Design review of the part built by this model. Coordinates are the model's own, in mm. A direction names the side the tool comes from. Give positions to 0.01 mm unless a question says otherwise; leave off trailing zeros. Write each loop counter-clockwise with the first axis right and the second up, starting at its lowest first coordinate (ties: lowest second). Pieces come first, ordered by that corner, then holes. Notation, with made-up numbers: (-2.5, 65) -> (18.5, 65) arc R33 ccw to (18.5, 100) -> close; hole circle Ø6 at (30.5, 66). An arc over 180 degrees is marked (long way). Return JSON: item names as keys, results as strings. Group by question number.
from build123d import *

# Parameters (mm, degrees)
F1_DEPTH = 10
F3_START = -8.5
F3_DEPTH = 1.5
F4_W     = 100
F4_H     = 3.1556577078
F5_DEPTH = 15
F6_R     = 2.1
F7_DEPTH = 3.1556577078


with BuildPart() as f1:
    # F0 (on Front) → F1 (new body)
    with BuildSketch(Plane.XZ):
        with BuildLine():
            Line((-40, 0), (0, 0))
            Line((0, 0), (40, 0))
            Line((40, 0), (39, 3))
            Line((39, 3), (7.4807440028, 74.4629067455))
            ThreePointArc((7.4807440028, 74.4629067455), (5.4899088977, 80.1098826107), (0, 82.5))
            ThreePointArc((0, 82.5), (-5.4899088977, 80.1098826107), (-7.4807440028, 74.4629067455))
            Line((-7.4807440028, 74.4629067455), (-39, 3))
            Line((-39, 3), (-40, 0))
        make_face()
        Polygon((-36.2676340608, 3), (-26.6060408243, 24.9055150458), (-11.2676340608, 3), align=None, mode=Mode.SUBTRACT)
        Polygon((-8.2156975889, 3), (-25.4265780732, 27.5796846579), (-1.5, 32.7676715966), (-1.5, 3), align=None, mode=Mode.SUBTRACT)
        Polygon((8.2156975889, 3), (1.5, 3), (1.5, 32.7676715966), (25.4265780732, 27.5796846579), align=None, mode=Mode.SUBTRACT)
        Polygon((26.6060408243, 24.9055150458), (36.2676340608, 3), (11.2676340608, 3), align=None, mode=Mode.SUBTRACT)
        Polygon((-14.0836967229, 53.2971467781), (-1.5, 35.3257653858), (-24.1790002431, 30.4082900711), align=None, mode=Mode.SUBTRACT)
        with BuildLine():
            Line((-1.5, 39.6843823749), (-12.9042339719, 55.9713163903))
            Line((-12.9042339719, 55.9713163903), (-6.3037586943, 70.9364269018))
            ThreePointArc((-6.3037586943, 70.9364269018), (-4.2334735249, 68.8090629212), (-1.5, 67.6515307717))
            Line((-1.5, 67.6515307717), (-1.5, 39.6843823749))
        make_face(mode=Mode.SUBTRACT)
        Polygon((1.5, 35.3257653858), (14.0836967229, 53.2971467781), (24.1790002431, 30.4082900711), align=None, mode=Mode.SUBTRACT)
        with BuildLine():
            Line((1.5, 39.6843823749), (1.5, 67.6515307717))
            ThreePointArc((1.5, 67.6515307717), (4.2334735249, 68.8090629212), (6.3037586943, 70.9364269018))
            Line((6.3037586943, 70.9364269018), (12.9042339719, 55.9713163903))
            Line((12.9042339719, 55.9713163903), (1.5, 39.6843823749))
        make_face(mode=Mode.SUBTRACT)
        with BuildLine():
            ThreePointArc((0, 80), (5, 75), (0, 70))
            ThreePointArc((0, 70), (-5, 75), (0, 80))
        make_face(mode=Mode.SUBTRACT)
    extrude(amount=F1_DEPTH)

    # F2 (on face) → F3 (join)
    with BuildSketch(Plane.XZ.offset(10).offset(F3_START)):
        Polygon((-1.5, 67.6515307717), (-7.4807440028, 74.4629067455), (-40, 0), (40, 0), (7.4807440028, 74.4629067455), (1.5, 67.6515307717), align=None)
    extrude(amount=-F3_DEPTH)

    # F4 (on Front) → F5 (join)
    with BuildSketch(Plane.XZ):
        with Locations((0, 1.5778288539)):
            Rectangle(F4_W, F4_H)
    extrude(amount=F5_DEPTH)

    # F6 (on face) → F7 (cut, through all)
    with BuildSketch(Plane.XY.offset(3.1556577078)):
        with Locations((-45, -7.5)):
            Circle(F6_R)
        with Locations((45, -7.5)):
            Circle(F6_R)
        with Locations((-25, -7.5)):
            Circle(F6_R)
        with Locations((25, -7.5)):
            Circle(F6_R)
    extrude(amount=-F7_DEPTH, mode=Mode.SUBTRACT)


solid = f1.part
Q1. Tool access review of faces 1 (the face through (0, -10, 37)), 2 (the face through (1.915, -4.93, 70.381)), 3 (the face through (19.06, -5.69, 42.01)): name each direction out of +Z, -Z, +X, -X, +Y, -Y from which nothing blocks a thin tool from reaching the whole face with its end or side.
Q2. Insertion check: pin 1 (5.5 mm diameter, centred on x = 25, y = -7.5, fed in from +Z); pin 2 (3.5 mm diameter, centred on x = 7, z = 57, fed in from -Y); pin 3 (12.5 mm diameter, centred on x = -8, z = 50, fed in from -Y). Each pin has a flat end and moves straight along its axis. Give the tip position at first contact, or say it passes through.
Q3. Take a section at A-A, the plane x = -45. Give the boundary of the cut face in (y, z).
Q4. Take a section at C-C, the plane y = -3.5. Count the separate pieces of the cut face and the enclosed holes in it, plus the area to 3 significant figures.
Q5. Take a section at B-B, the plane z = 66.5. Give the boundary of the cut face in (x, y).
Q6. Mouldability with a two-part tool opening along Z and no side actions: class faces 4 (the face through (23.426, -4.93, 38.31)), 5 (the face through (-11, -1.5, 18)), 6 (the face through (-43.87, -5.73, 1.6)), 7 (the face through (-1, -11, 3.156)) as +Z half, -Z half, draft (parallel to the pull), parting line (faces both ways), or undercut.
Q7. For L1, parallel to Y at x = -45, z = 2.25; L2, parallel to X at y = -3.75, z = 67; L3, parallel to X at y = -4, z = 49, list the stretches that pass through material, from the lowest coordinate up. Write a range as from..to.
Q8. Take a section at D-D, the plane y = -11.25. Give the boundary of the cut face in (x, z), plus the area to 3 significant figures.
Final values:
{
 "1": {"face 1": "+Z, +X, -X, -Y", "face 2": "+Y, -Y", "face 3": "-Y"},
 "2": {"pin 1": "stops at z = 40.98", "pin 2": "stops at y = -1.5", "pin 3": "stops at y = -10"},
 "3": {"outline": "(-15, 0) -> (-9.6, 0) -> (-9.6, 3.16) -> (-15, 3.16) -> close; (-5.4, 0) -> (0, 0) -> (0, 3.16) -> (-5.4, 3.16) -> close"},
 "4": {"separate pieces": "1", "enclosed holes": "9", "area": "1,350 mm²"},
 "5": {"outline": "(-10.99, -10) -> (-8.26, -10) -> (-8.26, -1.5) -> (-1.5, -1.5) -> (-1.5, -10) -> (1.5, -10) -> (1.5, -1.5) -> (8.26, -1.5) -> (8.26, -10) -> (10.99, -10) -> (10.99, 0) -> (-10.99, 0) -> close"},
 "6": {"face 4": "+Z half", "face 5": "undercut", "face 6": "draft", "face 7": "undercut"},
 "7": {"L1": "y = -15..-9.6, -5.4..0", "L2": "x = -10.77..-8.04, -1.5..1.5, 8.04..10.77", "L3": "x = -18.71..-15.98, -11.07..-8.02, -1.5..1.5, 8.02..11.07, 15.98..18.71"},
 "8": {"outline": "(-50, 0) -> (50, 0) -> (50, 3.16) -> (-50, 3.16) -> close", "area": "316 mm²"}
}
